Geometry: see drawing. Coordinates: mm, zero at the bounding-box minimum. A direction names the side the tool comes from. Give positions to 0.01 mm unless a question says otherwise; leave off trailing zeros. Write each loop counter-clockwise with the first axis right and the second up, starting at its lowest first coordinate (ties: lowest second). Pieces come first, ordered by that corner, then holes. Notation, with made-up numbers: (43.25, -32) -> (58.25, -32) arc R13 cw to (58.25, -23) -> close; hole circle Ø6 at (62.25, 37.5). An arc over 180 degrees is marked (long way). Answer as a JSON object with one key per item and string values. Group by question number.
Item 1: Access query for the marked faces 3, 4 and 5. Directions: +Z, -Z, +X, -X, +Y, -Y. A direction counts if a zero-diameter tool reaches every point of the face in a straight line with its end or side. Return the directions, or none.
Item 2: First-contact query: pin 1 Ø1.4 at (x, y) = (2.5, 6.5) entering from +Z; pin 2 Ø3 at (y, z) = (13.5, 3.5) entering from +X; pin 3 Ø1 at (y, z) = (2, 3.5) entering from +X (1 decimal). Flat tips, straight axial feed; report the tip coordinate or a pass-through.
Item 3: Section query C-C on z = 2.05. Return the cut outline in (x, y).
Item 4: Section query B-B on x = 10.7. Return the cut outline in (y, z), plus the area to 3 significant figures.
Item 5: Pull-direction query (X, two-part tool) for the marked faces 1 and 2; classes: pulls with the +X half, pulls with the -X half, needs draft (parallel to the pull), parting line crosses it, or undercut.
Item 6: Section query D-D on z = 4.2. Return the cut outline in (x, y), plus the area to 3 significant figures.
Item 7: Section query A-A on z = 0.9. Return the cut outline in (x, y), plus the area to 3 significant figures.
Item 8: Ray query, probe 1 along X at (y, z) = (8.25, 4.2); probe 2 along Z at (x, y) = (2.25, 6.75); probe 3 along X at (y, z) = (5.25, 2.15). Return the intervals inside material, ascending. Write a range as from..to.
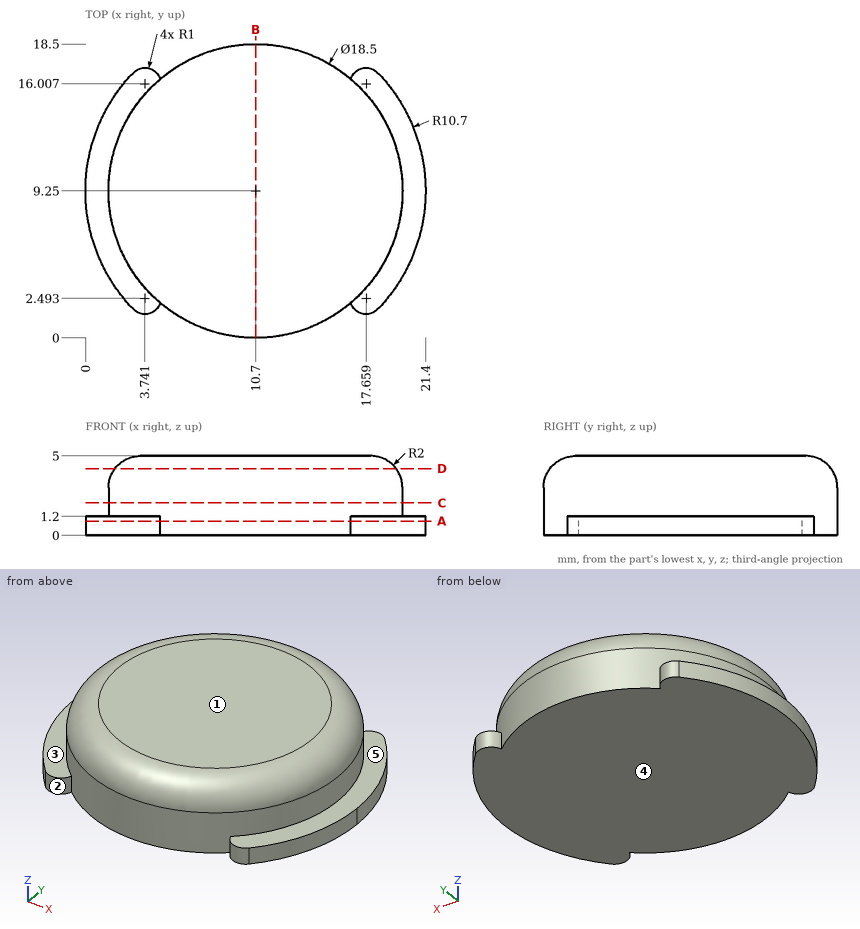
Worked answers:
{
 "1": {"face 3": "+Z, -X", "face 4": "-Z, +X, -X, +Y, -Y", "face 5": "+Z, +X"},
 "2": {"pin 1": "z = 4.87", "pin 2": "x = 19.51", "pin 3": "x = 17"},
 "3": {"outline": "circle Ø18.5 at (10.7, 9.25)"},
 "4": {"outline": "(0, 0) -> (18.5, 0) -> (18.5, 3) arc R2 ccw to (16.5, 5) -> (2, 5) arc R2 ccw to (0, 3) -> close", "area": "90.8 mm^2"},
 "5": {"face 1": "needs draft", "face 2": "undercut"},
 "6": {"outline": "circle Ø17.7 at (10.7, 9.25)", "area": "246 mm^2"},
 "7": {"outline": "(3.02, 1.8) arc R1 ccw to (4.7, 2.21) arc R9.25 ccw to (16.7, 2.21) arc R1 ccw to (18.38, 1.8) arc R10.7 ccw to (18.38, 16.7) arc R1 ccw to (16.7, 16.29) arc R9.25 ccw to (4.7, 16.29) arc R1 ccw to (3.02, 16.7) arc R10.7 ccw to start", "area": "318 mm^2"},
 "8": {"probe 1": "1.91..19.49", "probe 2": "0..4.25", "probe 3": "2.36..19.04"}
}
